Work out the finished part from the listing and answer in its coordinate system (mm). Face numbers are marked on the shaded views. Coordinates: 2 decimals unless noted, no trailing zeros. Order: outer loops, then holes, each group sorted by start corner. A loop starts at its lowest first (then second) coordinate and runs counter-clockwise, first axis right, second up.
```python
from build123d import *

# Parameters (mm, degrees)
SKETCH_4_W          = 50.742886584
SKETCH_4_H          = 35.769575788
EXTRUDE_3_DEPTH     = 20
CUT_EXTRUDE_1_DEPTH = 48
SKETCH_6_R          = 7.216894088
CUT_EXTRUDE_2_DEPTH = 68
SKETCH_7_W          = 16.696122742
SKETCH_7_H          = 32.152795324
CUT_EXTRUDE_4_DEPTH = 5
SKETCH_8_R          = 3.029228208
SKETCH_8_R_2        = 3.03
SKETCH_8_R_3        = 3.03083806
CUT_EXTRUDE_5_DEPTH = 3
SKETCH_9_W          = 5.030083898
SKETCH_9_H          = 0.631944611
SKETCH_9_W_2        = 7.178609771
SKETCH_9_H_2        = 0.710937687
SKETCH_9_W_3        = 7.570466712
EXTRUDE_5_DEPTH     = 48
SKETCH_10_W         = 27.632027184
SKETCH_10_H         = 0.724840375
SKETCH_10_H_2       = 0.710937687
SKETCH_10_H_3       = 0.631944611
EXTRUDE_6_DEPTH     = 48
SKETCH_13_W         = 1.627827619
SKETCH_13_H         = 35.769575788
EXTRUDE_9_DEPTH     = 20
SKETCH_15_W         = 1.627827619
SKETCH_15_H         = 32.092623512
EXTRUDE_11_DEPTH    = 20
SCALE_1_SCALE       = 2.16174


with BuildPart() as part:
    # 草图4 → 凸台-拉伸3 (new body)
    with BuildSketch(Plane(origin=(0, 0, 0), x_dir=(1, 0, 0), z_dir=(0, 1, 0))):
        Rectangle(SKETCH_4_W, SKETCH_4_H)
        with BuildLine():
            ThreePointArc((25.371443292, 17.884787894), (40.657584716, 0), (25.371443292, -17.884787894))
            Line((25.371443292, -17.884787894), (25.371443292, 17.884787894))
        make_face()
    extrude(amount=EXTRUDE_3_DEPTH)

    # 草图5 → 切除-拉伸1 (cut)
    with BuildSketch(Plane.ZY.offset(25.371443292)):
        with BuildLine():
            Line((-10.314321182, 17.711089067), (10.156549539, 17.711089067))
            ThreePointArc((10.156549539, 17.711089067), (17.33515931, 10.532479296), (10.156549539, 3.353869525))
            Line((10.156549539, 3.353869525), (-10.314321182, 3.353869525))
            ThreePointArc((-10.314321182, 3.353869525), (-17.492930953, 10.532479296), (-10.314321182, 17.711089067))
        make_face()
    extrude(amount=-CUT_EXTRUDE_1_DEPTH, mode=Mode.SUBTRACT)

    # 草图6 → 切除-拉伸2 (cut)
    with BuildSketch(Plane.ZY.offset(25.371443292)):
        with Locations((0, 10.493036385)):
            Circle(SKETCH_6_R)
    extrude(amount=-CUT_EXTRUDE_2_DEPTH, mode=Mode.SUBTRACT)

    # 草图7 → 切除-拉伸4 (cut)
    with BuildSketch(Plane(origin=(0, 20, 0), x_dir=(1, 0, 0), z_dir=(0, 1, 0))):
        with Locations((-15.177393996, 0.145817666)):
            Rectangle(SKETCH_7_W, SKETCH_7_H)
    extrude(amount=-CUT_EXTRUDE_4_DEPTH, mode=Mode.SUBTRACT)

    # 草图8 → 切除-拉伸5 (cut)
    with BuildSketch(Plane(origin=(0, 20, 0), x_dir=(1, 0, 0), z_dir=(0, 1, 0))):
        with Locations(Location((19.563664897, 0, 0), (0, 0, 270))):
            Circle(SKETCH_8_R)
        with Locations(Location((19.563664897, 8.712605536, 0), (0, 0, 270))):
            Circle(SKETCH_8_R_2)
        with Locations(Location((19.563664897, -8.858423201, 0), (0, 0, 270))):
            Circle(SKETCH_8_R_3)
    extrude(amount=-CUT_EXTRUDE_5_DEPTH, mode=Mode.SUBTRACT)

    # 草图9 → 凸台-拉伸5 (add)
    with BuildSketch(Plane.ZY.offset(25.371443292)):
        with Locations((-12.829363131, 16.299697839)):
            Rectangle(SKETCH_9_W, SKETCH_9_H)
        with Locations((-13.903626068, 13.929905549)):
            Rectangle(SKETCH_9_W_2, SKETCH_9_H_2)
        with Locations((-14.099554538, 11.402127105)):
            Rectangle(SKETCH_9_W_3, SKETCH_9_H_2)
    extrude(amount=-EXTRUDE_5_DEPTH)

    # 草图10 → 凸台-拉伸6 (add)
    with BuildSketch(Plane.ZY.offset(25.371443292)):
        with Locations((3.50169241, 11.395175762)):
            Rectangle(SKETCH_10_W, SKETCH_10_H)
        with Locations((3.50169241, 13.929905549)):
            Rectangle(SKETCH_10_W, SKETCH_10_H_2)
        with Locations((3.50169241, 16.299697839)):
            Rectangle(SKETCH_10_W, SKETCH_10_H_3)
    extrude(amount=-EXTRUDE_6_DEPTH)

    # 草图13 → 凸台-拉伸9 (add)
    with BuildSketch(Plane(origin=(0, 20, 0), x_dir=(1, 0, 0), z_dir=(0, 1, 0))):
        with Locations((-26.185357102, 0)):
            Rectangle(SKETCH_13_W, SKETCH_13_H)
    extrude(amount=-EXTRUDE_9_DEPTH)

    # 草图15 → 凸台-拉伸11 (add, through all)
    with BuildSketch(Plane(origin=(0, 20, 0), x_dir=(1, 0, 0), z_dir=(0, 1, 0))):
        with Locations((-26.185357102, 0.07480798)):
            Rectangle(SKETCH_15_W, SKETCH_15_H)
    extrude(amount=-EXTRUDE_11_DEPTH)


with BuildPart() as part_1:
    # 缩放比例1: scaled about (8.140035626, 9.333116532, 0.085734306)
    add(part.part.scale(SCALE_1_SCALE).moved(Location((-9.456604988, -10.8426548, -0.099600973))))


solid = part_1.part
```
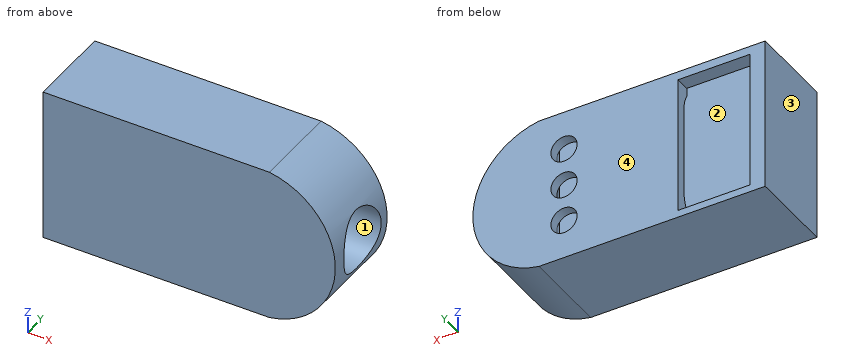
1. The part is cut by section D-D (y = 5). Determine the outline of the cut face in (x, z).
2. Flat-ended cylindrical pins translate along their axes: pin 1 (1.5 mm diameter, centred on x = 31, z = 18.5, fed in from +Y); pin 2 (0.8 mm diameter, centred on y = 14, z = -5.5, fed in from +X); pin 3 (5 mm diameter, centred on y = 12, z = -16, fed in from +X). Find the tip coordinate at first contact, or state that the pin passes through.
3. The part is cut by section B-B (x = 16.5). Count the separate pieces of the cut face and the enclosed holes in it, plus the area to 3 significant figures.
4. Consider probe 1 along Y at (x, z) = (-27, -23); probe 2 along Y at (x, z) = (31.5, -8.5); probe 3 along Z at (x, y) = (-55, 22.5). Determine where each line is inside the solid, lowest interval first.
5. The part is cut by section A-A (z = -20). Determine the outline of the cut face in (x, y), plus the area to 3 significant figures.
6. The mould has two halves that part along Y. Classify the marked faces 1, 2, 3 and 4: released by +Y, released by -Y, zero draft, split by the parting line, or undercut.
Worked out:
1. outline: (-67.82, -38.76) - (45.39, -38.76) arc R39.14 ccw to (75.84, -14.12) - (39.46, -14.12) - (39.46, -36.28) - (-64.3, -36.28) - (-64.3, 35.74) - (39.46, 35.74) - (39.46, 13.92) - (75.84, 13.92) arc R39.14 ccw to (45.39, 38.56) - (-67.82, 38.56) - close
2. pin 1: stops at y = 25.08
2. pin 2: stops at x = 39.46
2. pin 3: stops at x = 75.29
3. separate pieces: 1
3. enclosed holes: 4
3. area: 1,530 mm2
4. probe 1: y = -10.84 to -3.58, 13.04 to 14.57, 18.5 to 20.04, 23.71 to 25.08
4. probe 2: y = -10.84 to -3.59, 13.01 to 14.57, 18.5 to 20.04, 23.71 to 25.08, 27.44 to 32.39
4. probe 3: z = -38.76 to -35.17, 34.34 to 38.56
5. outline: (-67.82, -10.84) - (73, -10.84) - (73, 32.39) - (39.3, 32.39) - (39.3, 27.44) - (39.46, 27.44) - (39.46, 25.08) - (-64.3, 25.08) - (-64.3, 27.44) - (-60.31, 27.44) - (-60.31, 32.39) - (-67.82, 32.39) - close; (-24.22, 27.44) - (26.37, 27.44) - (26.37, 32.39) - (-24.22, 32.39) - close; hole (-64.3, -3.59) - (39.46, -3.59) - (39.46, 13.01) - (-64.3, 13.01) - close; hole (-64.3, 14.57) - (39.46, 14.57) - (39.46, 18.5) - (-64.3, 18.5) - close; hole (-64.3, 20.04) - (39.46, 20.04) - (39.46, 23.71) - (-64.3, 23.71) - close
5. area: 3,090 mm2
6. face 1: undercut
6. face 2: undercut
6. face 3: zero draft
6. face 4: released by +Y
